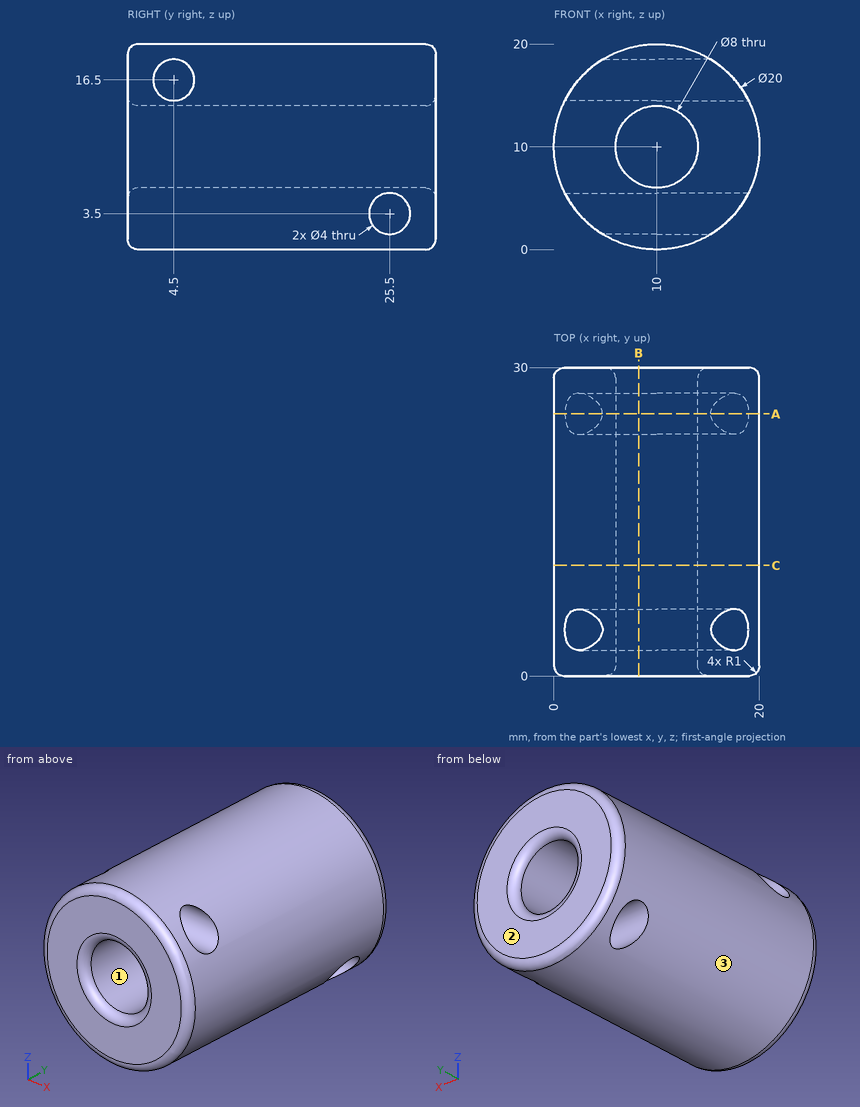
Geometry: see drawing. Coordinates: mm, zero at the bounding-box minimum. Coordinates: 2 decimals unless noted, no trailing zeros. Loops run counter-clockwise (first coordinate to the right, second up) from the corner with the lowest first, then second, coordinate; pieces in that order, holes last. Notation, with made-up numbers: (31, 25.5) -> (53, 25.5) arc R23 cw to (53, 53.5) -> close; hole circle Ø10 at (54.5, 26.25). An arc over 180 degrees is marked (long way). Use a Markdown table: item, result.
1) Cut plane A-A (y = 25.5). Return the cut outline in (x, z), then the cut area to 3 significant figures.
Results found:
| item | result |
|---|---|
| outline | (1.07, 5.5) -> (18.93, 5.5) arc R10 ccw (long way) to start; (4.73, 1.5) arc R10 ccw to (15.27, 1.5) -> close; hole circle Ø8 at (10, 10) |
| area | 204 mm2 |
2) Contact query for flat-ended pins moving along their axis: pin 1 (1 mm diameter, centred on x = 16, z = 9, fed in from -Y); pin 2 (1.5 mm diameter, centred on x = 14, y = 22.5, fed in from -Z); pin 3 (3 mm diameter, centred on x = 16, y = 6.5, fed in from +Z); pin 4 (8 mm diameter, centred on y = 8.5, z = 15, fed in from -X). Output: stop coordinate, or through.
Results found:
| item | result |
|---|---|
| pin 1 | stops at y = 0 |
| pin 2 | stops at z = 0.54 |
| pin 3 | stops at z = 18.93 |
| pin 4 | stops at x = 0.05 |
3) Pull-direction query (X, two-part tool) for the marked faces 1, 2 and 3; classes: released by +X, released by -X, zero draft, split by the parting line, or undercut.
Results found:
| item | result |
|---|---|
| face 1 | undercut |
| face 2 | zero draft |
| face 3 | split by the parting line |
4) Cut plane B-B (x = 8.25). Give the number of separate pieces and of enclosed holes in the cut face, then the cut area to 3 significant figures.
Results found:
| item | result |
|---|---|
| separate pieces | 2 |
| enclosed holes | 2 |
| area | 348 mm2 |
5) Material intervals for line 1 along Y through (x, z) = (13.25, 3.5); line 2 along Z through (x, y) = (11, 2.75); line 3 along Y through (x, z) = (5, 16.5), sorted ascending. Write a range as from..to.
Results found:
| item | result |
|---|---|
| line 1 | y = 0..23.5, 27.5..30 |
| line 2 | z = 0.05..6.13, 13.87..15.53, 17.47..19.95 |
| line 3 | y = 0..2.5, 6.5..30 |
6) Cut plane C-C (y = 10.75). Return the cut outline in (x, z).
Results found:
| item | result |
|---|---|
| outline | circle Ø20 at (10, 10); hole circle Ø8 at (10, 10) |
